The figure shows three views and two pictorial views of one solid part (mm, origin at its lowest corner). Answer the questions. Coordinates: 2 decimals unless noted, no trailing zeros. Write each loop counter-clockwise with the first axis right and the second up, starting at its lowest first coordinate (ties: lowest second). Pieces come first, ordered by that corner, then holes.
Item 1: Section A-A (x = 114.3) is taken. Give the vertices of the cut face in (y, z) (1 decimal), then the cut area to 3 significant figures.
Item 2: Section D-D (z = 165.1) is taken. Give the vertices of the cut face in (x, y) (1 decimal), then the cut area to 3 significant figures.
Item 3: Straight lines are drawn through the part: probe 1 along Z at (x, y) = (114.3, 1.6); probe 2 along X at (y, z) = (2, 76.2); probe 3 along X at (y, z) = (1.15, 139.7). For each, find the intervals that lie inside material, in ascending order.
Item 4: This flat-tipped pin is pushed along its axis until it touches: P1, Ø2.5, axis at x = 114.3, z = 165.1, coming from the -Y side. Where does it stop, or does it pass through?
Item 5: Section B-B (z = 12.7) is taken. Give the vertices of the cut face in (x, y) (1 decimal).
Item 6: Section C-C (x = 12.7) is taken. Give the vertices of the cut face in (y, z) (1 decimal).
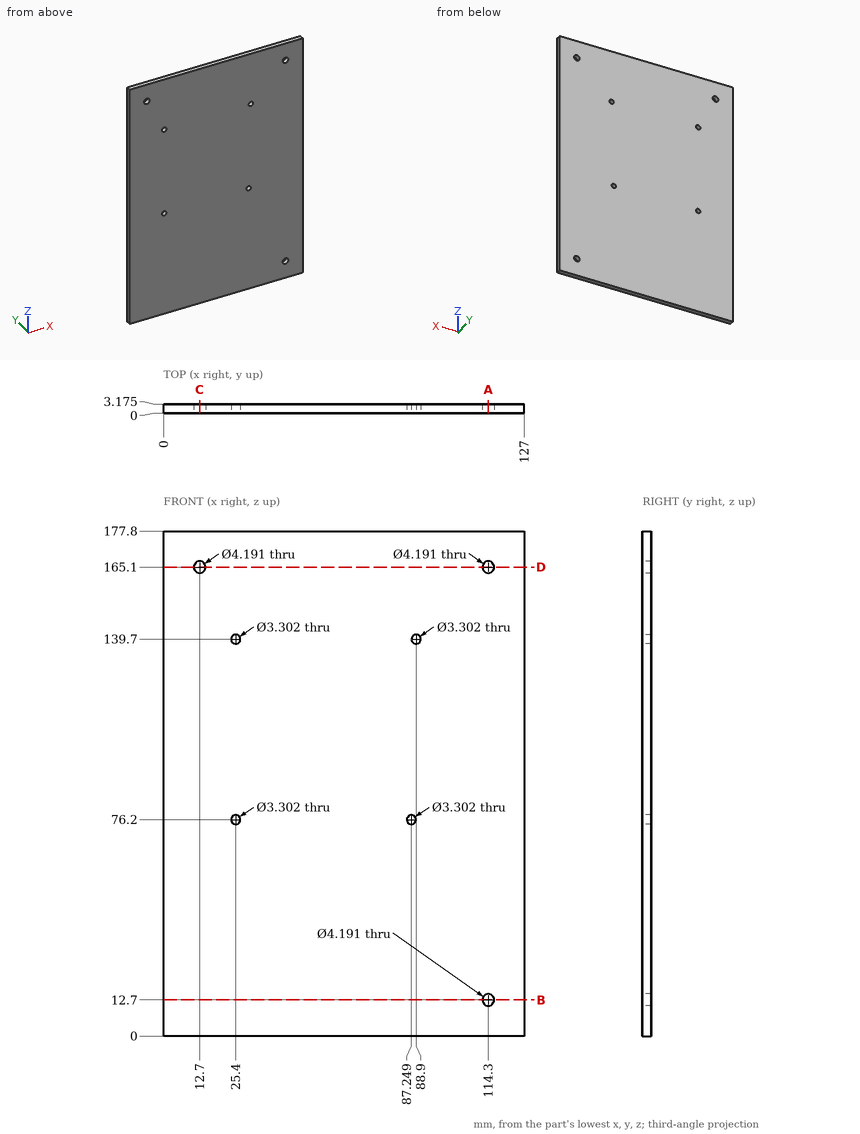
Established:
1. outline: (0, 0) - (3.2, 0) - (3.2, 10.6) - (0, 10.6) - close; (0, 14.8) - (3.2, 14.8) - (3.2, 163) - (0, 163) - close; (0, 167.2) - (3.2, 167.2) - (3.2, 177.8) - (0, 177.8) - close
1. area: 538 mm2
2. outline: (0, 0) - (10.6, 0) - (10.6, 3.2) - (0, 3.2) - close; (14.8, 0) - (112.2, 0) - (112.2, 3.2) - (14.8, 3.2) - close; (116.4, 0) - (127, 0) - (127, 3.2) - (116.4, 3.2) - close
2. area: 377 mm2
3. probe 1: z = 0 to 10.6, 14.8 to 163, 167.2 to 177.8
3. probe 2: x = 0 to 23.75, 27.05 to 85.6, 88.9 to 127
3. probe 3: x = 0 to 23.75, 27.05 to 87.25, 90.55 to 127
4. P1: passes through
5. outline: (0, 0) - (112.2, 0) - (112.2, 3.2) - (0, 3.2) - close; (116.4, 0) - (127, 0) - (127, 3.2) - (116.4, 3.2) - close
6. outline: (0, 0) - (3.2, 0) - (3.2, 163) - (0, 163) - close; (0, 167.2) - (3.2, 167.2) - (3.2, 177.8) - (0, 177.8) - close
